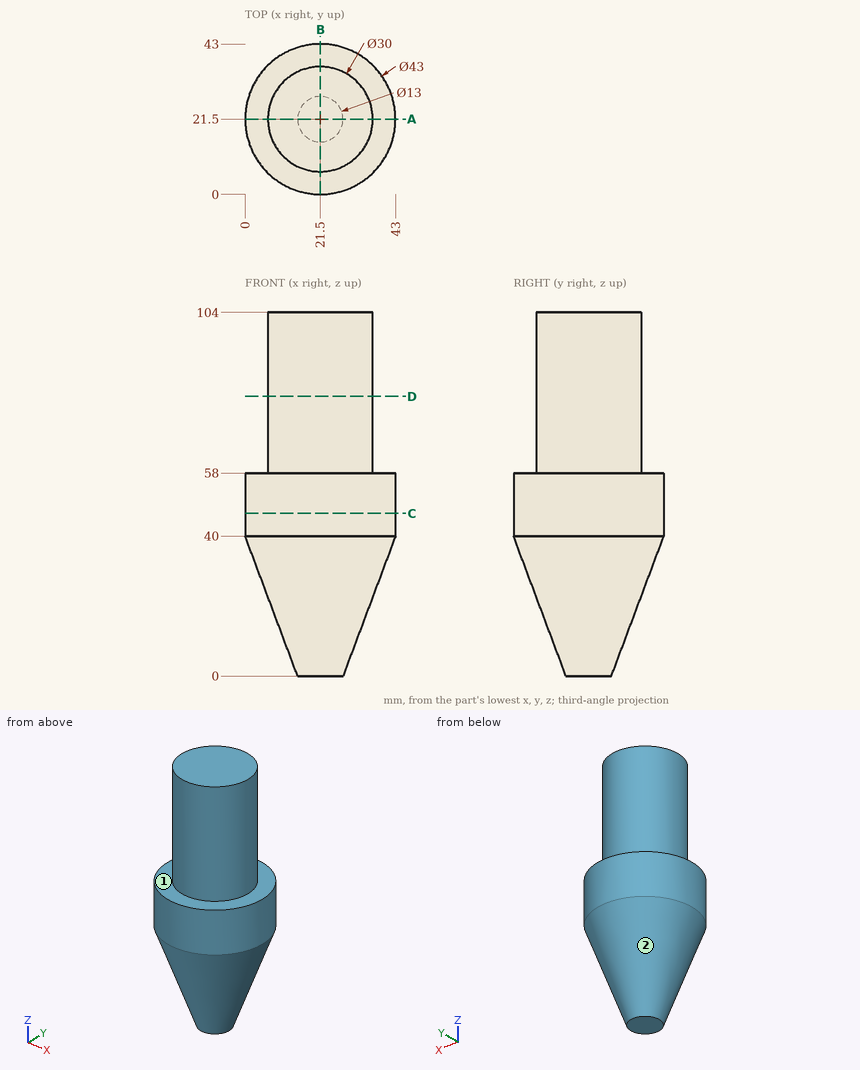
Design review of the part shown in the three views and the two pictorial views. Dimensions are in mm from the part's minimum x, y and z. A direction names the side the tool comes from. Round coordinates to 2 decimals unless told otherwise and drop trailing zeros. Write each loop counter-clockwise with the first axis right and the second up, starting at its lowest first coordinate (ties: lowest second). Pieces come first, ordered by that corner, then holes. Notation, with made-up numbers: (26, -22.5) - (62, -22.5) arc R15 ccw to (62, -9.5) - close; hole circle Ø10 at (10, 85.5). An arc over 180 degrees is marked (long way). Return JSON: item names as keys, results as strings. Group by question number.
Item 1: For probe 1 along Y at (x, z) = (24.5, 7); probe 2 along Y at (x, z) = (8, 92); probe 3 along Z at (x, y) = (36, 29), list the stretches that pass through material, from the lowest coordinate up. Write a range as [from, to].
Item 2: We need section D-D on z = 80. Write out the cut boundary in (x, y), and give its area (3 significant figures).
Item 3: Machinability: for the marked faces 1 and 2, which of the approach directions +Z, -Z, +X, -X, +Y, -Y give a long, thin tool a straight path to every point of the face, cutting with its end or side? Answer none if there is none.
Item 4: We need section A-A on y = 21.5. Write out the cut boundary in (x, z).
Item 5: Insertion check: P1, Ø3, axis at x = 17, z = 16, coming from the -Y side; P2, Ø5, axis at y = 10.5, z = 54, coming from the +X side; P3, Ø4, axis at y = 11.5, z = 64.5, coming from the +X side. Each pin has a flat end and moves straight along its axis. Give the tip position at first contact, or say it passes through.
Item 6: We need section C-C on z = 46.5. Write out the cut boundary in (x, y).
Model answer:
{
 "1": {"probe 1": "y = [12.88, 30.12]", "probe 2": "y = [14.96, 28.04]", "probe 3": "z = [26.2, 58]"},
 "2": {"outline": "circle Ø30 at (21.5, 21.5)", "area": "707 mm²"},
 "3": {"face 1": "+Z", "face 2": "-Z"},
 "4": {"outline": "(0, 40) - (15, 0) - (28, 0) - (43, 40) - (43, 58) - (36.5, 58) - (36.5, 104) - (6.5, 104) - (6.5, 58) - (0, 58) - close"},
 "5": {"P1": "stops at y = 9.06", "P2": "stops at x = 41.25", "P3": "stops at x = 34.19"},
 "6": {"outline": "circle Ø43 at (21.5, 21.5)"}
}
